Can you work these out from the model? Positions are in its coordinate system, mm. Coordinates: 2 decimals unless noted, no trailing zeros. Order: outer loops, then holes, each group sorted by start corner. A loop starts at its lowest first (then second) coordinate and runs counter-clockwise, first axis right, second up.
```python
from build123d import *

# Parameters (mm, degrees)
ESQUISSE1_R      = 12
ESQUISSE1_R_2    = 1.5
ESQUISSE1_R_3    = 2.5
EXTRUSION1_DEPTH = 2
CHANFREIN1_SIZE  = 0.5


with BuildPart() as part:
    # Esquisse1 → Extrusion1 (new body)
    with BuildSketch(Plane(origin=(0, 0, 0), x_dir=(1, 0, 0), z_dir=(0, 1, 0))):
        with BuildLine():
            Line((-25, -2.5), (-21.742814905, -2.5))
            ThreePointArc((-21.742814905, -2.5), (-18.840417096, -3.428625913), (-17.016116013, -5.869565217))
            ThreePointArc((-17.016116013, -5.869565217), (17.365780251, -4.735997916), (-11.680287305, 13.695652174))
            ThreePointArc((-11.680287305, 13.695652174), (-13.19590137, 12.808425684), (-14.924811557, 12.5))
            Line((-14.924811557, 12.5), (-25, 12.5))
            ThreePointArc((-25, 12.5), (-32.5, 5), (-25, -2.5))
        make_face()
        Circle(ESQUISSE1_R, mode=Mode.SUBTRACT)
        with Locations((-12.557368355, -7.25)):
            Circle(ESQUISSE1_R_2, mode=Mode.SUBTRACT)
        with Locations((12.557368355, -7.25)):
            Circle(ESQUISSE1_R_2, mode=Mode.SUBTRACT)
        with Locations((0, 14.5)):
            Circle(ESQUISSE1_R_2, mode=Mode.SUBTRACT)
        with Locations((-25, 5)):
            Circle(ESQUISSE1_R_3, mode=Mode.SUBTRACT)
    extrude(amount=EXTRUSION1_DEPTH)

    # Chanfrein1
    chanfrein1_edges = [part.edges().sort_by_distance(p)[0] for p in [
        (-12, 0, 0),
        (-12, 2, 0),
    ]]
    chamfer(chanfrein1_edges, length=CHANFREIN1_SIZE)


solid = part.part
```
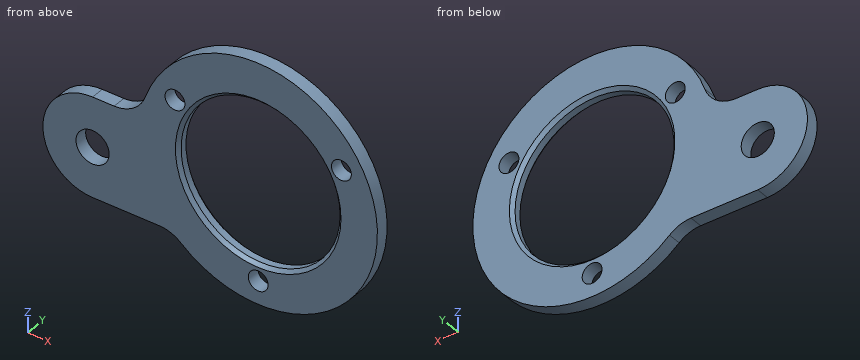
1. Imagine slicing it at B-B on z = -14.5. Please give me the cut outline in (x, y).
Completed:
outline: (-10.67, 0) - (-1.5, 0) - (-1.5, 2) - (-10.67, 2) - close; (1.5, 0) - (10.67, 0) - (10.67, 2) - (1.5, 2) - close
2. Please list where these lines run through material, in increasing order: probe 1 along Z at (x, y) = (0, 1.15); probe 2 along Z at (x, y) = (1, 0.25); probe 3 along X at (y, z) = (0.4, -4).
Completed:
probe 1: z = -18 to -16, -13 to -12, 12 to 18
probe 2: z = -17.97 to -15.62, -13.38 to -12.21, 12.21 to 17.97
probe 3: x = -32.43 to -27.29, -22.71 to -11.42, 11.42 to 17.55
3. Imagine slicing it at C-C on z = 7.25. Give the number of separate pieces and of enclosed holes in the cut face, then the cut area to 3 significant figures.
Completed:
separate pieces: 4
enclosed holes: 0
area: 15.0 mm2
4. I'm going to push flat-ended pins straight in: pin 1 (1 mm diameter, centred on x = -27, y = 1.5, fed in from +Z); pin 2 (1 mm diameter, centred on x = -22.5, y = 1, fed in from +Z). Where does each tip first touch, or does it pass through?
Completed:
pin 1: stops at z = 2.35
pin 2: stops at z = 2.5
5. Imagine slicing it at A-A on y = 0.95. Please give me the cut outline in (x, z), then the cut area to 3 significant figures.
Completed:
outline: (-25, -12.5) - (-14.92, -12.5) arc R5 cw to (-11.68, -13.7) arc R18 ccw (long way) to (-17.02, 5.87) arc R5 cw to (-21.74, 2.5) - (-25, 2.5) arc R7.5 ccw to start; hole circle Ø5 at (-25, -5); hole circle Ø3 at (-12.56, 7.25); hole circle Ø24 at (0, 0); hole circle Ø3 at (0, -14.5); hole circle Ø3 at (12.56, 7.25)
area: 741 mm2
